from build123d import *

# Parameters (mm, degrees)
SKETCH1_W           = 70
SKETCH1_H           = 15
BOSS_EXTRUDE1_DEPTH = 1
SKETCH2_W           = 5
SKETCH2_H           = 15
BOSS_EXTRUDE2_DEPTH = 11
SKETCH3_R           = 1.6
CUT_EXTRUDE1_DEPTH  = 8
SKETCH4_W           = 5.5
SKETCH4_H           = 3
CUT_EXTRUDE2_DEPTH  = 72.416034614


with BuildPart() as part:
    # Sketch1 → Boss-Extrude1 (new body)
    with BuildSketch(Plane(origin=(0, 0, 0), x_dir=(1, 0, 0), z_dir=(0, 1, 0))):
        Rectangle(SKETCH1_W, SKETCH1_H)
    extrude(amount=BOSS_EXTRUDE1_DEPTH)

    # Sketch2 → Boss-Extrude2 (add)
    with BuildSketch(Plane(origin=(0, 1, 0), x_dir=(1, 0, 0), z_dir=(0, 1, 0))):
        with Locations((-32.5, 0)):
            Rectangle(SKETCH2_W, SKETCH2_H)
        with Locations((32.5, 0)):
            Rectangle(SKETCH2_W, SKETCH2_H)
    extrude(amount=BOSS_EXTRUDE2_DEPTH)

    # Sketch3 → Cut-Extrude1 (cut)
    with BuildSketch(Plane(origin=(0, 12, 0), x_dir=(1, 0, 0), z_dir=(0, 1, 0))):
        with Locations(Location((-32.5, 0, 0), (0, 0, 270))):
            Circle(SKETCH3_R)
        with Locations(Location((32.5, 0, 0), (0, 0, 90))):
            Circle(SKETCH3_R)
    extrude(amount=-CUT_EXTRUDE1_DEPTH, mode=Mode.SUBTRACT)

    # Sketch4 → Cut-Extrude2 (cut, through all)
    with BuildSketch(Plane(origin=(35, 0, 0), x_dir=(0, 0, -1), z_dir=(1, 0, 0))):
        with Locations((0, 6.5)):
            Rectangle(SKETCH4_W, SKETCH4_H)
    extrude(amount=-CUT_EXTRUDE2_DEPTH, mode=Mode.SUBTRACT)


solid = part.part
CAD build for the part. Positions are in the model's coordinates, mm. A direction names the side the tool comes from. Round coordinates to 2 decimals unless told otherwise and drop trailing zeros. Loops run counter-clockwise (first coordinate to the right, second up) from the corner with the lowest first, then second, coordinate; pieces in that order, holes last.
(1) Cut at C-C (x = -32.5). Give the cut face in (y, z).
(2) Cut at A-A (y = 11.25). Give the cut face in (x, z).
(3) Which spindle directions (+Z, -Z, +X, -X, +Y, -Y) get a long thin tool onto all of the face, cutting with end or side? Do faces 4 (the flat face through (-35, 4.6, 0.1)), 5 (the cylindrical face through (33.92, 10.03, -0.74)), 6 (the flat face through (33, 6, 2.75)), 7 (the flat face through (0, 0, 0)), 8 (the flat face through (0, 1, 0)). Say none if no direction does.
(4) Cut at B-B (z = 0). State how many separate pieces and enclosed holes the cut face has, plus the area to 3 significant figures.
(5) Wall check: line 1 along X through (y, z) = (4.8, 0); line 2 along X through (y, z) = (9.5, 3.25); line 3 along Z through (x, y) = (32.5, 4.45). Give the ranges that are in metal, low to high.
(6) Drop a flat-ended pin along its axis: pin 1 (1 mm diameter, centred on x = 32.5, z = 0.5, fed in from +Y). Give the stop position or say it passes through.
(7) Two-plate mould, pull along X, no slides. Class faces 1 (the flat face through (35, 4.6, 0.1)), 2 (the flat face through (-32, 6, 2.75)), 3 (the cylindrical face through (-33.92, 10.03, 0.74)): +X half, -X half, draft (parallel to the pull), parting line (faces both ways), or undercut.
(8) Cut at D-D (z = 5.25). Give the cut face in (x, y), plus the area to 3 significant figures.
Findings below:
1. outline: (0, -7.5) - (12, -7.5) - (12, -1.6) - (8, -1.6) - (8, -2.75) - (5, -2.75) - (5, -1.6) - (4, -1.6) - (4, 1.6) - (5, 1.6) - (5, 2.75) - (8, 2.75) - (8, 1.6) - (12, 1.6) - (12, 7.5) - (0, 7.5) - close
2. outline: (-35, -7.5) - (-30, -7.5) - (-30, 7.5) - (-35, 7.5) - close; (30, -7.5) - (35, -7.5) - (35, 7.5) - (30, 7.5) - close; hole circle Ø3.2 at (-32.5, 0); hole circle Ø3.2 at (32.5, 0)
3. face 4: +Z, -Z, -X, +Y, -Y
3. face 5: +Y
3. face 6: +X, -X
3. face 7: +Z, -Z, +X, -X, -Y
3. face 8: +Z, -Z, +Y
4. separate pieces: 5
4. enclosed holes: 0
4. area: 118 mm2
5. line 1: x = -35 to -34.1, -30.9 to -30, 30 to 30.9, 34.1 to 35
5. line 2: x = -35 to -30, 30 to 35
5. line 3: z = -7.5 to -1.6, 1.6 to 7.5
6. pin 1: stops at y = 4
7. face 1: +X half
7. face 2: draft
7. face 3: undercut
8. outline: (-35, 0) - (35, 0) - (35, 12) - (30, 12) - (30, 1) - (-30, 1) - (-30, 12) - (-35, 12) - close
8. area: 180 mm2
